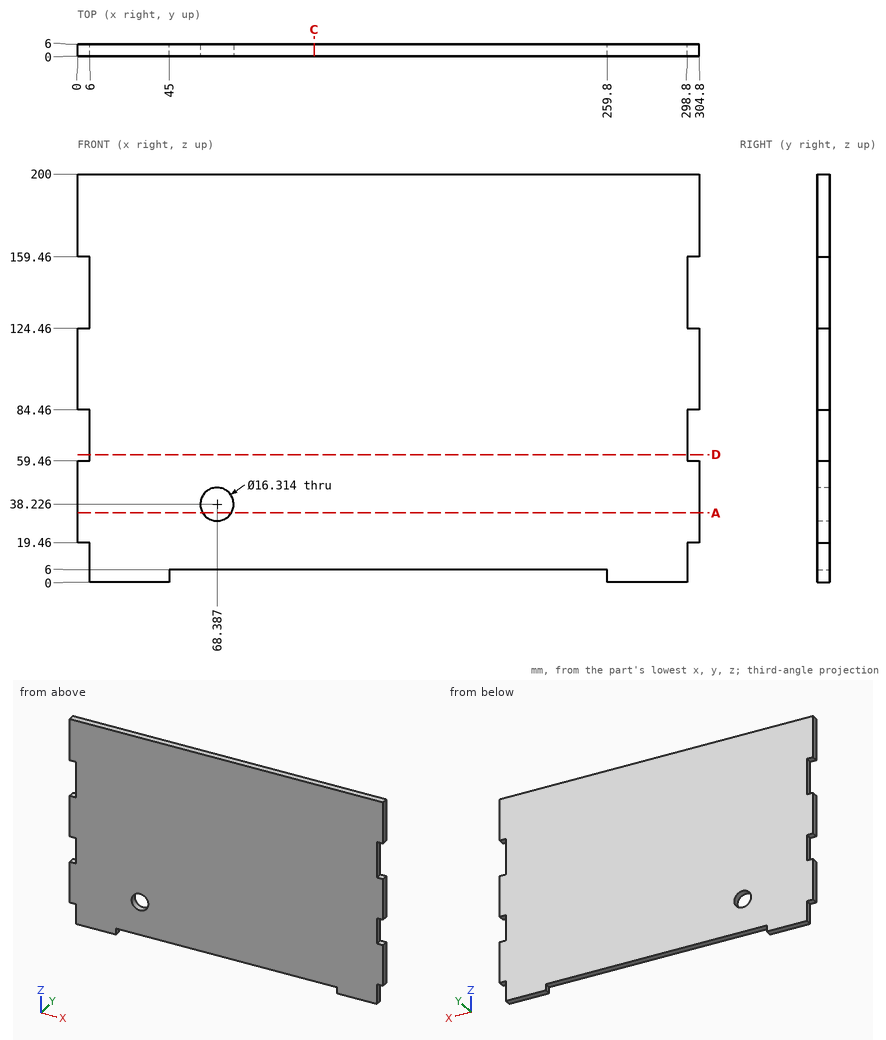
Source: three-view drawing plus pictorial views. Frame: mm from the lowest corner of the part. Round coordinates to 2 decimals unless told otherwise and drop trailing zeros. Loops run counter-clockwise (first coordinate to the right, second up) from the corner with the lowest first, then second, coordinate; pieces in that order, holes last.
1. Section query C-C on x = 116. Output: boundary loops of the cut face in (y, z), and give its area (3 significant figures).
2. Ray query, L1, parallel to X at y = 4.8, z = 66; L2, parallel to Z at x = 205, y = 2.75. Return the intervals inside material, ascending.
3. Section query A-A on z = 34. Output: boundary loops of the cut face in (x, y), and give its area (4 significant figures).
4. Contact query for flat-ended pins moving along their axis: pin 1 (3 mm diameter, centred on x = 3, y = 3, fed in from -Z); pin 2 (1.8 mm diameter, centred on y = 4, z = 1.5, fed in from -X); pin 3 (1.5 mm diameter, centred on x = 60.5, z = 144, fed in from -Y); pin 4 (1.8 mm diameter, centred on y = 3.5, z = 67, fed in from +X). Output: stop coordinate, or through.
5. Section query D-D on z = 62.5. Output: boundary loops of the cut face in (x, y), and give its area (3 significant figures).
Answers below:
1. outline: (0, 6) - (6, 6) - (6, 200) - (0, 200) - close
1. area: 1,160 mm2
2. L1: x = 6 to 298.8
2. L2: z = 6 to 200
3. outline: (0, 0) - (61.41, 0) - (61.41, 6) - (0, 6) - close; (75.36, 0) - (304.8, 0) - (304.8, 6) - (75.36, 6) - close
3. area: 1,745 mm2
4. pin 1: stops at z = 19.46
4. pin 2: stops at x = 6
4. pin 3: stops at y = 0
4. pin 4: stops at x = 298.8
5. outline: (6, 0) - (298.8, 0) - (298.8, 6) - (6, 6) - close
5. area: 1,760 mm2
